Geometry: final body of the model. Coordinates: model frame, mm. A direction names the side the tool comes from. Round coordinates to 2 decimals unless told otherwise and drop trailing zeros. Order: outer loops, then holes, each group sorted by start corner. A loop starts at its lowest first (then second) coordinate and runs counter-clockwise, first axis right, second up. Notation, with made-up numbers: (24, -22) -> (78, -22) arc R27 cw to (78, 4) -> close; hole circle Ø3 at (62, 41.25). An arc over 180 degrees is marked (long way). Put each result on its own line as item: value.
```python
from build123d import *

# Parameters (mm, degrees)
BOSS_EXTRUDE1_START = 9.525
SKETCH3_R           = 12.7
SKETCH3_R_2         = 6.3627
BOSS_EXTRUDE1_DEPTH = 3.175
BOSS_EXTRUDE2_START = 6.35
SKETCH4_R           = 9.5504
SKETCH4_R_2         = 6.3627
BOSS_EXTRUDE2_DEPTH = 15.875
CHAMFER1_SIZE       = 0.190881


with BuildPart() as part:
    # Sketch3 → Boss-Extrude1 (new body)
    with BuildSketch(Plane.XY.offset(BOSS_EXTRUDE1_START)):
        Circle(SKETCH3_R)
        Circle(SKETCH3_R_2, mode=Mode.SUBTRACT)
    extrude(amount=-BOSS_EXTRUDE1_DEPTH)

    # Sketch4 → Boss-Extrude2 (add)
    with BuildSketch(Plane.XY.offset(BOSS_EXTRUDE2_START)):
        Circle(SKETCH4_R)
        Circle(SKETCH4_R_2, mode=Mode.SUBTRACT)
    extrude(amount=-BOSS_EXTRUDE2_DEPTH)

    # Chamfer1
    chamfer1_edges = [part.edges().sort_by_distance(p)[0] for p in [
        (-6.3627, 0, -9.525),
        (-9.5504, 0, 6.35),
        (-12.7, 0, 9.525),
        (-12.7, 0, 6.35),
        (-6.3627, 0, 9.525),
        (-9.5504, 0, -9.525),
    ]]
    chamfer(chamfer1_edges, length=CHAMFER1_SIZE)


solid = part.part
```
1. Material intervals for probe 1 along Y at (x, z) = (0, 0); probe 2 along Z at (x, y) = (1.25, -9.75) (3 decimals); probe 3 along Y at (x, z) = (-3, 3), sorted ascending.
Ans:
probe 1: -9.55 to -6.36, 6.36 to 9.55
probe 2: 6.35 to 9.525
probe 3: -9.07 to -5.61, 5.61 to 9.07
2. Cut plane C-C on z = -7.5. Return loops of the section in (x, y), and give its area (3 significant figures).
Ans:
outline: circle Ø19.1 at (0, 0); hole circle Ø12.73 at (0, 0)
area: 159 mm²
3. Contact query for flat-ended pins moving along their axis: P1, Ø5, axis at x = -2.5, z = 0.5, coming from the +Y side; P2, Ø1, axis at x = -2.5, z = -4.5, coming from the +Y side; P3, Ø10, axis at x = 10, z = 3, coming from the -Y side. Output: stop coordinate, or through.
Ans:
P1: y = 9.55
P2: y = 9.34
P3: y = -10.93
4. Draft query along Y for faces 1 (the face through (-0.83, 6.31, 0.13)), 2 (the face through (-2.07, -9.323, -1.479)), 3 (the face through (5, -5, 9.525)). Return one class per face: +Y half, -Y half, draft (parallel to the pull), parting line (faces both ways), or undercut.
Ans:
face 1: undercut
face 2: parting line
face 3: draft
5. Set-up query: faces 4 (the face through (-2.75, -12.4, 7.96)), 5 (the face through (0, -10, 6.35)). Return all of +Z, -Z, +X, -X, +Y, -Y with unobstructed straight access to the full face (end or side cutting, diameter ignored); none if empty.
Ans:
face 4: +Z, -Z
face 5: -Z
6. Cut plane A-A on x = 0. Return loops of the section in (y, z) (3 decimals), and give its area (3 significant figures).
Ans:
outline: (-12.7, 6.541) -> (-12.509, 6.35) -> (-9.741, 6.35) -> (-9.55, 6.159) -> (-9.55, -9.334) -> (-9.36, -9.525) -> (-6.554, -9.525) -> (-6.363, -9.334) -> (-6.363, 9.334) -> (-6.554, 9.525) -> (-12.509, 9.525) -> (-12.7, 9.334) -> close; (6.363, -9.334) -> (6.554, -9.525) -> (9.36, -9.525) -> (9.55, -9.334) -> (9.55, 6.159) -> (9.741, 6.35) -> (12.509, 6.35) -> (12.7, 6.541) -> (12.7, 9.334) -> (12.509, 9.525) -> (6.554, 9.525) -> (6.363, 9.334) -> close
area: 141 mm²
